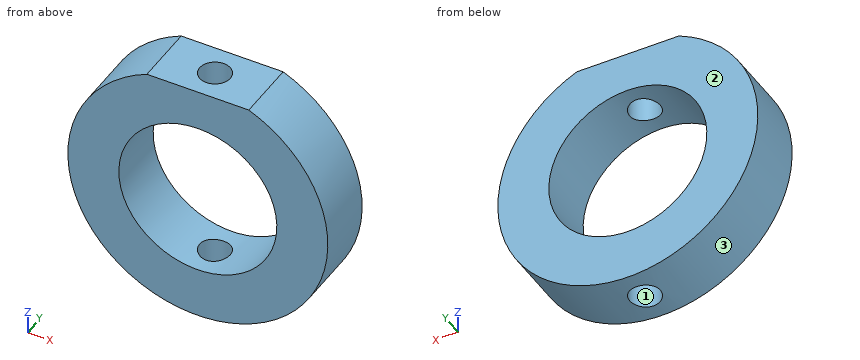
from build123d import *

# Parameters (mm, degrees)
SKETCH1_R           = 7.75
BOSS_EXTRUDE1_DEPTH = 6
SKETCH2_R           = 1.5
CUT_EXTRUDE1_DEPTH  = 29.244812881


with BuildPart() as part:
    # Sketch1 → Boss-Extrude1 (new body)
    with BuildSketch(Plane(origin=(0, 0, 0), x_dir=(1, 0, 0), z_dir=(0, 1, 0))):
        with BuildLine():
            Line((-5, -11.728704106), (5, -11.728704106))
            ThreePointArc((5, -11.728704106), (0, 12.75), (-5, -11.728704106))
        make_face()
        with Locations(Location((0, 0, 0), (0, 0, 270))):
            Circle(SKETCH1_R, mode=Mode.SUBTRACT)
    extrude(amount=BOSS_EXTRUDE1_DEPTH)

    # Sketch2 → Cut-Extrude1 (cut, through all)
    with BuildSketch(Plane.XY.offset(11.728704106)):
        with Locations((0, 3)):
            Circle(SKETCH2_R)
    extrude(amount=-CUT_EXTRUDE1_DEPTH, mode=Mode.SUBTRACT)


solid = part.part
Part model, mm, in its own coordinate system. Face numbers are marked on the shaded views. Coordinates: 2 decimals unless noted, no trailing zeros. Loops run counter-clockwise (first coordinate to the right, second up) from the corner with the lowest first, then second, coordinate; pieces in that order, holes last. Notation, with made-up numbers: M -23,88 L 34,88 A28 ccw 34,123 Z; hole C 64,3 d5. An arc over 180 degrees is marked long. Use a Markdown table: item, result. Add a question column.
Q1. Probe L1, parallel to Y at x = 0, z = -9.95; L2, parallel to X at y = 4.75, z = 0; L3, parallel to X at y = 3, z = -2. List the from-to ranges inside material, lowest first.
Q2. Cut at C-C (y = 3). Write the cut outline in (x, z), and give its area (3 significant figures).
Q3. Cut at A-A (x = 0). Write the cut outline in (y, z).
Q4. Pin check, flat tips, straight feed: P1, Ø2.5, axis at x = 0, y = 3, coming from the -Z side; P2, Ø1, axis at x = 9.5, y = 3, coming from the -Z side. Stop position of each tip, or through.
Q5. Mould opens along X. For the marked faces 1, 2 and 3 say: +X half, -X half, draft (parallel to the pull), parting line (faces both ways), or undercut.
Q6. Cut at B-B (z = 0). Write the cut outline in (x, y).
Q7. Cut at D-D (x = -3.5). Write the cut outline in (y, z).
Worked out:
| question | item | result |
|---|---|---|
| 1 | L1 | y = 0 to 1.5, 4.5 to 6 |
| 1 | L2 | x = -12.75 to -7.75, 7.75 to 12.75 |
| 1 | L3 | x = -12.59 to -7.49, 7.49 to 12.59 |
| 2 | outline | M -5,11.73 A12.75 ccw -1.5,-12.66 L -1.5,-7.6 A7.75 cw -1.5,7.6 L -1.5,11.73 Z; M 1.5,-12.66 A12.75 ccw 5,11.73 L 1.5,11.73 L 1.5,7.6 A7.75 cw 1.5,-7.6 Z |
| 2 | area | 288 mm2 |
| 3 | outline | M 0,-12.75 L 1.5,-12.75 L 1.5,-7.75 L 0,-7.75 Z; M 0,7.75 L 1.5,7.75 L 1.5,11.73 L 0,11.73 Z; M 4.5,-12.75 L 6,-12.75 L 6,-7.75 L 4.5,-7.75 Z; M 4.5,7.75 L 6,7.75 L 6,11.73 L 4.5,11.73 Z |
| 4 | P1 | passes through |
| 4 | P2 | stops at z = -9.03 |
| 5 | face 1 | undercut |
| 5 | face 2 | draft |
| 5 | face 3 | parting line |
| 6 | outline | M -12.75,0 L -7.75,0 L -7.75,6 L -12.75,6 Z; M 7.75,0 L 12.75,0 L 12.75,6 L 7.75,6 Z |
| 7 | outline | M 0,-12.26 L 6,-12.26 L 6,-6.91 L 0,-6.91 Z; M 0,6.91 L 6,6.91 L 6,11.73 L 0,11.73 Z |
